Can you work these out from the drawing? Everything is in mm from the part's minimum corner. Coordinates: 2 decimals unless noted, no trailing zeros. Loops run counter-clockwise (first coordinate to the right, second up) from the corner with the lowest first, then second, coordinate; pieces in that order, holes last.
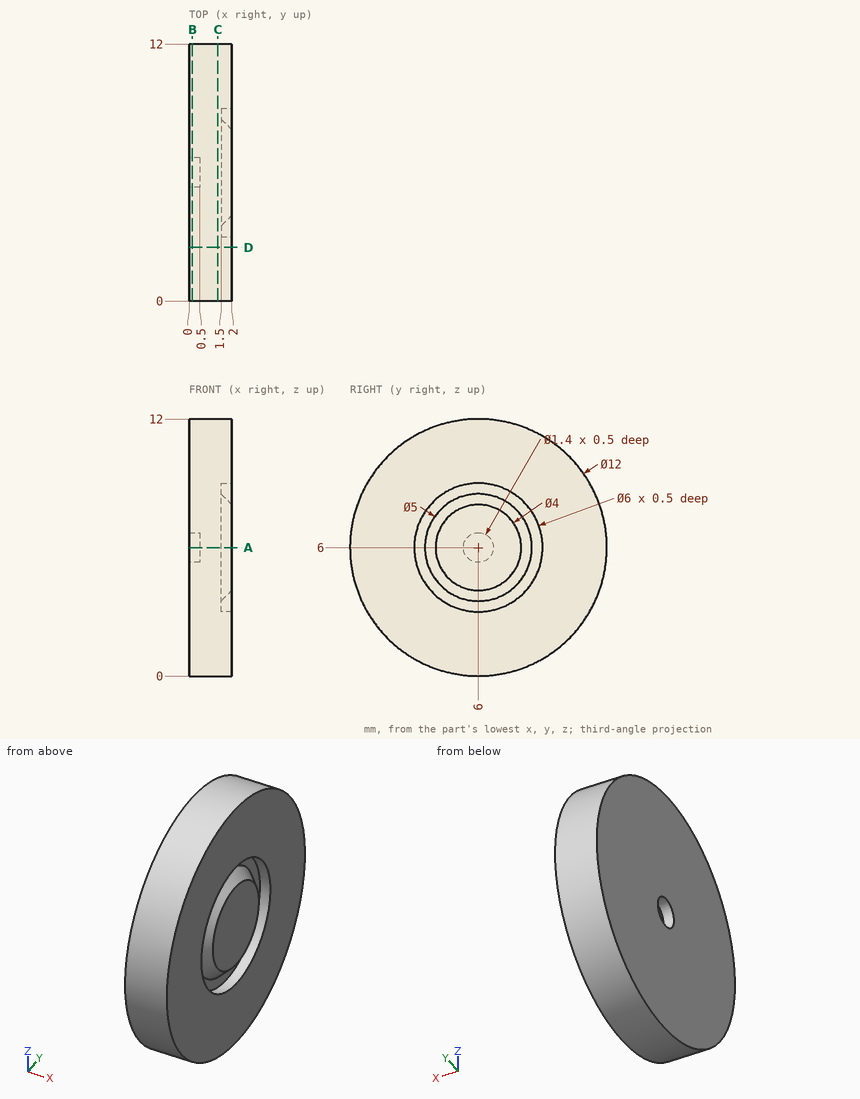
(1) Imagine slicing it at D-D, the plane y = 2.5. Write out the boundary of the cut face in (x, z), and give its area (3 significant figures).
Answers:
outline: (0, 1.13) - (2, 1.13) - (2, 10.87) - (0, 10.87) - close
area: 19.5 mm2
(2) I need wall thicknesses on probe 1 along Y at (x, z) = (0.1, 6); probe 2 along Y at (x, z) = (1.9, 5.5); probe 3 along Y at (x, z) = (1.55, 8). Which ranges of each line are inside material? Lowest first, please.
Answers:
probe 1: y = 0 to 5.3, 6.7 to 12
probe 2: y = 0.02 to 3.04, 3.96 to 8.04, 8.96 to 11.98
probe 3: y = 0.34 to 3.76, 4.58 to 7.42, 8.24 to 11.66
(3) Imagine slicing it at B-B, the plane x = 0.15. Write out the boundary of the cut face in (y, z), and give its area (3 significant figures).
Answers:
outline: circle Ø12 at (6, 6); hole circle Ø1.4 at (6, 6)
area: 112 mm2
(4) Imagine slicing it at A-A, the plane z = 6. Write out the boundary of the cut face in (x, y).
Answers:
outline: (0, 0) - (2, 0) - (2, 3) - (1.5, 3) - (1.5, 3.5) - (2, 4) - (2, 8) - (1.5, 8.5) - (1.5, 9) - (2, 9) - (2, 12) - (0, 12) - (0, 6.7) - (0.5, 6.7) - (0.5, 5.3) - (0, 5.3) - close
(5) For pin 1 (1.6 mm diameter, centred on y = 6, z = 6, fed in from -X); pin 2 (1 mm diameter, centred on x = 1.5, y = 2, fed in from +Z); pin 3 (1.1 mm diameter, centred on y = 6, z = 6, fed in from -X), each with a flat end and sliding along its axis, tell me the tip position at first contact or that it passes through.
Answers:
pin 1: stops at x = 0
pin 2: stops at z = 10.87
pin 3: stops at x = 0.5
(6) Imagine slicing it at C-C, the plane x = 1.35. Write out the boundary of the cut face in (y, z).
Answers:
outline: circle Ø12 at (6, 6)
